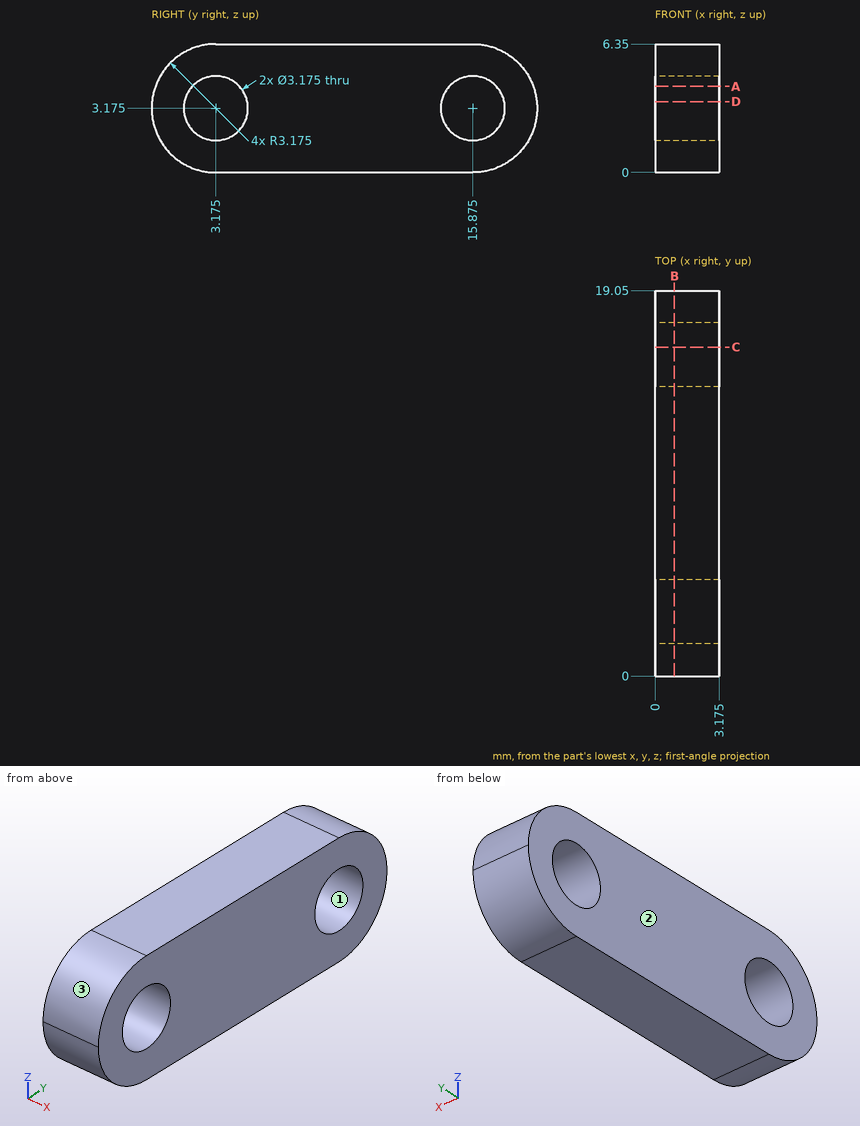
For this review, use the dimensioned drawing (mm, ordinates from the lowest corner) and the shaded views. Coordinates: 2 decimals unless noted, no trailing zeros. Loops run counter-clockwise (first coordinate to the right, second up) from the corner with the lowest first, then second, coordinate; pieces in that order, holes last. Notation, with made-up numbers: (73, -36) -> (104, -36) arc R35 ccw to (104, -3) -> close; hole circle Ø5 at (43.5, 88). An arc over 180 degrees is marked (long way). Use a Markdown table: item, result. Add a question column.
1. Add section C-C on y = 16.25. Write out the cut boundary in (x, z) (1 decimal), plus the area to 3 significant figures.
2. Add section A-A on z = 4.25. Write out the cut boundary in (x, y) (1 decimal).
3. Add section B-B on x = 0.95. Give the number of separate pieces and of enclosed holes in the cut face, plus the area to 3 significant figures.
4. Add section D-D on z = 3.5. Write out the cut boundary in (x, y) (1 decimal).
5. Draft analysis for pull direction Z (two halves, no side actions). For the marked faces 1, 2 and 3, state which applies: pulls with the +Z half, pulls with the -Z half, needs draft (parallel to the pull), parting line crosses it, or undercut.
6. To check wall thickness, follow line 1 (Y direction, x = 2.45, z = 3.5); line 2 (Y direction, x = 2.4, z = 1.75) (1 decimal); line 3 (Z direction, x = 0.25, y = 15). State the ranges of each line that lie inside material, in increasing order.
Returned:
| question | item | result |
|---|---|---|
| 1 | outline | (0, 0) -> (3.2, 0) -> (3.2, 1.6) -> (0, 1.6) -> close; (0, 4.7) -> (3.2, 4.7) -> (3.2, 6.3) -> (0, 6.3) -> close |
| 1 | area | 10.2 mm² |
| 2 | outline | (0, 0.2) -> (3.2, 0.2) -> (3.2, 2) -> (0, 2) -> close; (0, 4.3) -> (3.2, 4.3) -> (3.2, 14.7) -> (0, 14.7) -> close; (0, 17) -> (3.2, 17) -> (3.2, 18.9) -> (0, 18.9) -> close |
| 3 | separate pieces | 1 |
| 3 | enclosed holes | 2 |
| 3 | area | 96.5 mm² |
| 4 | outline | (0, 0) -> (3.2, 0) -> (3.2, 1.6) -> (0, 1.6) -> close; (0, 4.7) -> (3.2, 4.7) -> (3.2, 14.3) -> (0, 14.3) -> close; (0, 17.4) -> (3.2, 17.4) -> (3.2, 19) -> (0, 19) -> close |
| 5 | face 1 | undercut |
| 5 | face 2 | needs draft |
| 5 | face 3 | pulls with the +Z half |
| 6 | line 1 | y = 0.02 to 1.62, 4.73 to 14.32, 17.43 to 19.03 |
| 6 | line 2 | y = 0.3 to 2.5, 3.9 to 15.2, 16.6 to 18.7 |
| 6 | line 3 | z = 0 to 1.85, 4.5 to 6.35 |
